Check sheet for the modelled part. Datum: model origin and axes. Units: mm. A direction names the side the tool comes from. Round coordinates to 2 decimals unless told otherwise and drop trailing zeros. Write each loop counter-clockwise with the first axis right and the second up, starting at its lowest first coordinate (ties: lowest second). Pieces come first, ordered by that corner, then holes.
from build123d import *

# Parameters (mm, degrees)
SKETCH_1_R          = 50
EXTRUDE_1_DEPTH     = 20
SKETCH_2_R          = 45
CUT_EXTRUDE_1_DEPTH = 8
SKETCH_3_R          = 44
CUT_EXTRUDE_2_DEPTH = 12
CHAMFER_1_SIZE      = 1


with BuildPart() as part:
    # 스케치1 → 보스-돌출1 (new body)
    with BuildSketch(Plane.XY):
        Circle(SKETCH_1_R)
    extrude(amount=EXTRUDE_1_DEPTH)

    # 스케치2 → 컷-돌출1 (cut)
    with BuildSketch(Plane.XY.offset(20)):
        Circle(SKETCH_2_R)
    extrude(amount=-CUT_EXTRUDE_1_DEPTH, mode=Mode.SUBTRACT)

    # 스케치3 → 컷-돌출2 (cut)
    with BuildSketch(Plane(origin=(0, 0, 0), x_dir=(-1, 0, 0), z_dir=(0, 0, -1))):
        Circle(SKETCH_3_R)
    extrude(amount=-CUT_EXTRUDE_2_DEPTH, mode=Mode.SUBTRACT)

    # 모따기1
    chamfer_1_edges = [part.edges().sort_by_distance(p)[0] for p in [
        (44, 0, 0),
        (-50, 0, 0),
        (-50, 0, 20),
        (-45, 0, 20),
    ]]
    chamfer(chamfer_1_edges, length=CHAMFER_1_SIZE)


solid = part.part
1. Sectioned sample at D-D, the plane z = 5. Enter the section's corners in (x, y).
2. Release check for a two-part mould opening along X. For faces 1 (the flat face through (22, -40, 0)), 2 (the cylindrical face through (47.69, 15.02, 9.87)), 3 (the cylindrical face through (20.765, -39.923, 15.549)), 4 (the cylindrical face through (9.538, -42.954, 6.423)) record: released by +X, released by -X, zero draft, split by the parting line, or undercut.
3. Sectioned sample at A-A, the plane y = 0. Enter the section's corners in (x, z).
4. Go/stop test with flat-tipped pins: pin 1 (1 mm diameter, centred on y = 26.5, z = 7.5, fed in from +X); pin 2 (4 mm diameter, centred on y = 31, z = 13.5, fed in from +X); pin 3 (4 mm diameter, centred on y = 27.5, z = 11.5, fed in from -X). Record where each tip stops, or that it passes through.
5. Scan lines: line 1 along X through (y, z) = (1.5, 18) (1 decimal); line 2 along Y through (x, z) = (1, 10.25). Record each from-to range of solid material in increasing order.
6. Sectioned sample at C-C, the plane z = 16.5. Enter the section's corners in (x, y).
7. Set-up check for faces 5 (the flat face through (43.1, -9.8, 12)), 6 (the flat face through (14, 44, 20)): record each of +Z, -Z, +X, -X, +Y, -Y from which the full face is reachable in a straight line by a thin tool's end or side.
Computed values:
1. outline: circle Ø100 at (0, 0); hole circle Ø88 at (0, 0)
2. face 1: zero draft
2. face 2: split by the parting line
2. face 3: undercut
2. face 4: undercut
3. outline: (-50, 1) - (-49, 0) - (-45, 0) - (-44, 1) - (-44, 12) - (-45, 12) - (-45, 19) - (-46, 20) - (-49, 20) - (-50, 19) - close; (44, 1) - (45, 0) - (49, 0) - (50, 1) - (50, 19) - (49, 20) - (46, 20) - (45, 19) - (45, 12) - (44, 12) - close
4. pin 1: stops at x = 42.71
4. pin 2: stops at x = 40.73
4. pin 3: stops at x = -43.01
5. line 1: x = -50 to -45, 45 to 50
5. line 2: y = -49.99 to -43.99, 43.99 to 49.99
6. outline: circle Ø100 at (0, 0); hole circle Ø90 at (0, 0)
7. face 5: +Z
7. face 6: +Z, +X, -X, +Y, -Y
